from build123d import *

# Parameters (mm, degrees)
SKETCH_1_R          = 2.5
EXTRUDE_1_DEPTH     = 41.8
SKETCH_6_R          = 1.1
CUT_EXTRUDE_1_DEPTH = 1


with BuildPart() as part:
    # 草图1 → 凸台-拉伸1 (new body)
    with BuildSketch(Plane(origin=(0, 0, 0), x_dir=(1, 0, 0), z_dir=(0, 1, 0))):
        Circle(SKETCH_1_R)
    extrude(amount=EXTRUDE_1_DEPTH)

    # 草图6 → 切除-拉伸1 (cut)
    with BuildSketch(Plane(origin=(2.5, 0, 0), x_dir=(0, 0, -1), z_dir=(1, 0, 0))):
        with Locations((0, 39.3)):
            Circle(SKETCH_6_R)
        with Locations((0, 2.5)):
            Circle(SKETCH_6_R)
    extrude(amount=-CUT_EXTRUDE_1_DEPTH, mode=Mode.SUBTRACT)


solid = part.part
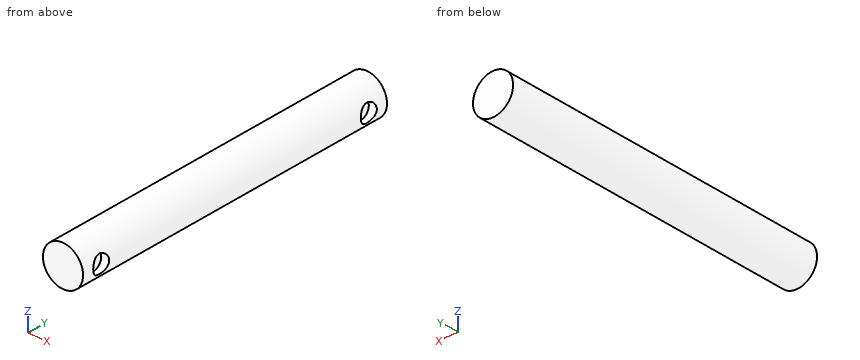
The model under review builds one solid part; all positions refer to its coordinate system, in mm. Round coordinates to 2 decimals unless told otherwise and drop trailing zeros. Order: outer loops, then holes, each group sorted by start corner. A loop starts at its lowest first (then second) coordinate and runs counter-clockwise, first axis right, second up. Notation, with made-up numbers: (29.5, 40) -> (83.5, 40) arc R28 ccw to (83.5, 74) -> close; hole circle Ø1 at (0, -22). An arc over 180 degrees is marked (long way). Use CSV: the item, a comma, the result in double quotes. Start each with the question number.
(1) Consider section D-D on z = -1.5. Write out the cut boundary in (x, y), and give its area (3 significant figures).
(2) Wall thickness on probe 1 along Y at (x, z) = (1.8, 0); probe 2 along Z at (x, y) = (-0.2, 16.5); probe 3 along Z at (x, y) = (2.1, 2.5): over which ranges is each line inside the solid? List them lowest first. Write a range as from..to.
(3) Insertion check: pin 1 (0.7 mm diameter, centred on y = 39.5, z = 0, fed in from +X); pin 2 (1.5 mm diameter, centred on y = 7.5, z = -2, fed in from -X); pin 3 (2 mm diameter, centred on y = 5, z = 1.5, fed in from +X). Each pin has a flat end and moves straight along its axis. Give the tip position at first contact, or say it passes through.
(4) Consider section C-C on x = -1.55. Write out the cut boundary in (y, z).
(5) Consider section A-A on z = 0.55. Write out the cut boundary in (x, y), and give its area (3 significant figures).
(6) Consider section B-B on y = 18. Write out the cut boundary in (x, z).
Responses:
1,outline,"(-2, 0) -> (2, 0) -> (2, 41.8) -> (-2, 41.8) -> close"
1,area,"167 mm²"
2,probe 1,"0..1.4, 3.6..38.2, 40.4..41.8"
2,probe 2,"-2.49..2.49"
2,probe 3,"-1.36..-1.1, 1.1..1.36"
3,pin 1,"x = 1.5"
3,pin 2,"x = -2.17"
3,pin 3,"x = 2.45"
4,outline,"(0, -1.96) -> (41.8, -1.96) -> (41.8, 1.96) -> (0, 1.96) -> close"
5,outline,"(-2.44, 0) -> (2.44, 0) -> (2.44, 1.55) -> (1.5, 1.55) -> (1.5, 3.45) -> (2.44, 3.45) -> (2.44, 38.35) -> (1.5, 38.35) -> (1.5, 40.25) -> (2.44, 40.25) -> (2.44, 41.8) -> (-2.44, 41.8) -> close"
5,area,"200 mm²"
6,outline,"circle Ø5 at (0, 0)"
